Source: CAD feature listing. Evaluate the final solid. Frame: model axes, mm. Give positions to 0.01 mm unless a question says otherwise; leave off trailing zeros.
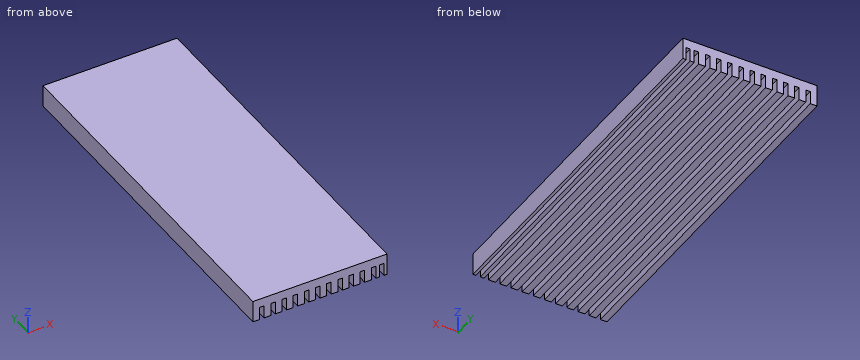
```python
from build123d import *

# Parameters (mm, degrees)
EXTRUDE_1_DEPTH = 160


with BuildPart() as part:
    # Эскиз1 → Бобышка-Вытянуть1 (new body)
    with BuildSketch(Plane(origin=(0, 0, 0), x_dir=(1, 0, 0), z_dir=(0, 1, 0))):
        Polygon((-30, 0), (30, 0), (30, 9.81929979), (28.644603918, 9.81929979), (28.644603918, 4), (26.747359492, 4), (26.747359492, 9.81929979), (25, 9.81929979), (25, 4), (23, 4), (23, 9.81929979), (20, 9.81929979), (20, 4), (18, 4), (18, 9.81929979), (15, 9.81929979), (15, 4), (13, 4), (13, 9.81929979), (10, 9.81929979), (10, 4), (8, 4), (8, 9.81929979), (5, 9.81929979), (5, 4), (3, 4), (3, 9.81929979), (0, 9.81929979), (0, 4), (-2, 4), (-2, 9.81929979), (-5, 9.81929979), (-5, 4), (-7, 4), (-7, 9.81929979), (-10, 9.81929979), (-10, 4), (-12, 4), (-12, 9.81929979), (-15, 9.81929979), (-15, 4), (-17, 4), (-17, 9.81929979), (-20, 9.81929979), (-20, 4), (-22, 4), (-22, 9.81929979), (-25, 9.81929979), (-25, 4), (-27, 4), (-27, 9.81929979), (-30, 9.81929979), align=None)
    extrude(amount=EXTRUDE_1_DEPTH)


solid = part.part
```
(1) Section A-A, the plane z = -7.75. Count the separate pieces of the cut face and the enclosed holes in it, then the cut area to 3 significant figures.
A:
separate pieces: 13
enclosed holes: 0
area: 5,780 mm2
(2) First-contact query: pin 1 (0.6 mm diameter, centred on x = -6.5, y = 61.5, fed in from -Z). Flat tip, straight axial feed; report the tip coordinate or a pass-through.
A:
pin 1: stops at z = -4
(3) Ray query, line 1 along Z through (x, y) = (9.5, 133). Return the intervals inside material, ascending.
A:
line 1: z = -4 to 0
